The listing builds one solid part. Answer for the finished solid, in the listing's coordinates (mm). Face numbers are marked on the shaded views. A direction names the side the tool comes from. Round coordinates to 2 decimals unless told otherwise and drop trailing zeros. Write each loop counter-clockwise with the first axis right and the second up, starting at its lowest first coordinate (ties: lowest second). Pieces come first, ordered by that corner, then holes.
(1) A cutting plane is placed at A-A, the plane x = 0. Give the vertices of the cut face in (y, z) (3 decimals).
(2) A cutting plane is placed at B-B, the plane y = -16.5. Give the vertices of the cut face in (x, z).
(3) Each of these flat-tipped pins is pushed along its axis until it touches: pin 1 Ø3 at (y, z) = (0, 5) entering from +X (3 decimals); pin 2 Ø6 at (y, z) = (-4.5, 3) entering from -X; pin 3 Ø5.5 at (x, y) = (-9.9, -9.9) entering from +Z; pin 4 Ø2 at (x, y) = (9.9, -9.9) entering from +Z. Where does it stop, or does it pass through?
(4) For the marked faces 1, 2, 3 and 4, determine the directions among +Z, -Z, +X, -X, +Y, -Y from which every point of the face is accessible in a straight line to the end or side of a thin tool.
(5) Find the intervals of material crossed by probe 1 along Y at (x, z) = (0, 6.25) (3 decimals); probe 2 along X at (y, z) = (34.25, 5); probe 3 along X at (y, z) = (-34.5, 5), in increasing order.
(6) The mould has two halves that part along Z. Classify the marked faces 5, 6 and 7: +Z half, -Z half, draft (parallel to the pull), parting line (faces both ways), or undercut.
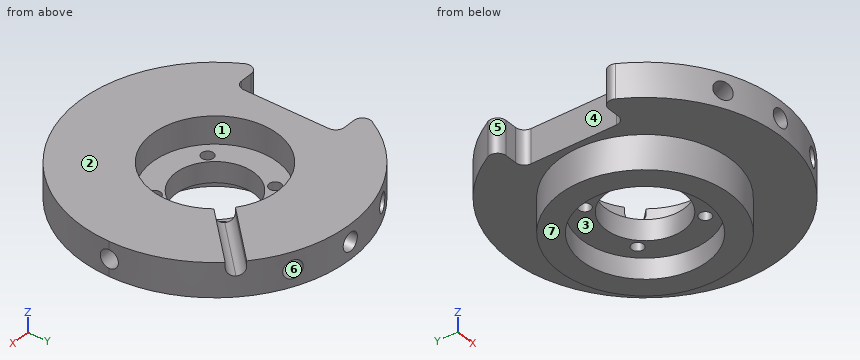
from build123d import *

# Parameters (mm, degrees)
SKETCH_1_R                = 39.675
EXTRUDE_1_DEPTH           = 10
SKETCH_7_R                = 2.65
CUT_EXTRUDE_5_DEPTH       = 8
PATTERN_CIRCULAR_1_COUNT  = 2
PATTERN_CIRCULAR_1_ANGLE  = 25
F_1_THE_OTHER_WAY_COUNT   = 2
F_1_THE_OTHER_WAY_ANGLE   = 25
MIRROR_1_COPY_1_SKETCH_R  = 2.65
MIRROR_1_COPY_1_DEPTH     = 8
MIRROR_1_COPY_2_SKETCH_R  = 2.65
MIRROR_1_COPY_2_DEPTH     = 8
SKETCH_9_R                = 2.65
CUT_EXTRUDE_7_DEPTH       = 8
PATTERN_CIRCULAR_2_COUNT  = 2
CUT_EXTRUDE_START         = -10
CUT_EXTRUDE_8_DEPTH       = 10
CUT_EXTRUDE_13_DEPTH      = 4
SKETCH_12_R               = 25
EXTRUDE_2_DEPTH           = 10
CUT_EXTRUDE_16_DEPTH      = 57.993080877
CUT_EXTRUDE_16_DEPTH_BACK = 57.993080877
SKETCH_18_R               = 11.5
SKETCH_18_R_2             = 1.75
SKETCH_19_R               = 18.4
CUT_EXTRUDE_17_DEPTH      = 6
CUT_EXTRUDE_START_2       = -8
SKETCH_20_R               = 18.4
CUT_EXTRUDE_18_DEPTH      = 8
FILLET_2_R                = 2.5


# Read off the part's stored shape, not the designer's step: Вырез-Вытянуть8
with BuildPart() as part:
    # Эскиз1 → Бобышка-Вытянуть1 (new body)
    with BuildSketch(Plane.XY):
        Circle(SKETCH_1_R)
    extrude(amount=EXTRUDE_1_DEPTH)

    # Эскиз7 → Вырез-Вытянуть5 (cut)
    with BuildSketch(Plane(origin=(0, 39.675, 0), x_dir=(0, 0, -1), z_dir=(0, 1, 0))):
        with Locations(Location((-5, 0, 0), (0, 0, 90))):
            Circle(SKETCH_7_R)
    cut_extrude_5 = extrude(amount=-CUT_EXTRUDE_5_DEPTH, mode=Mode.SUBTRACT)

    # Круговой массив1: Вырез-Вытянуть5 ×2 about axis
    pattern_circular_1_axis = Axis((0, 0, 10), (0, 0, -1))
    for i in range(1, PATTERN_CIRCULAR_1_COUNT):
        add(cut_extrude_5.rotate(pattern_circular_1_axis, i * PATTERN_CIRCULAR_1_ANGLE / (PATTERN_CIRCULAR_1_COUNT - 1)), mode=Mode.SUBTRACT)

    # 1 the other way: Вырез-Вытянуть5 ×2 about axis
    f_1_the_other_way_axis = Axis((0, 0, 10), (0, 0, 1))
    for i in range(1, F_1_THE_OTHER_WAY_COUNT):
        add(cut_extrude_5.rotate(f_1_the_other_way_axis, i * F_1_THE_OTHER_WAY_ANGLE / (F_1_THE_OTHER_WAY_COUNT - 1)), mode=Mode.SUBTRACT)

    # Зеркальное отражение1: Вырез-Вытянуть5 across plane
    add(cut_extrude_5.mirror(Plane.ZX), mode=Mode.SUBTRACT)

    # Зеркальное отражение1 copy 1 sketch → Зеркальное отражение1 copy 1 (cut)
    with BuildSketch(Plane(origin=(16.767379535, -35.957761451, 0), x_dir=(0, 0, -1), z_dir=(0.4226182617407035, -0.906307787036648, 0))):
        with Locations((-5, 0)):
            Circle(MIRROR_1_COPY_1_SKETCH_R)
    extrude(amount=-MIRROR_1_COPY_1_DEPTH, mode=Mode.SUBTRACT)

    # Зеркальное отражение1 copy 2 sketch → Зеркальное отражение1 copy 2 (cut)
    with BuildSketch(Plane(origin=(-16.767379535, -35.957761451, 0), x_dir=(0, 0, -1), z_dir=(-0.42261826174069717, -0.9063077870366509, 0))):
        with Locations((-5, 0)):
            Circle(MIRROR_1_COPY_2_SKETCH_R)
    extrude(amount=-MIRROR_1_COPY_2_DEPTH, mode=Mode.SUBTRACT)

    # Эскиз9 → Вырез-Вытянуть7 (cut)
    with BuildSketch(Plane.ZY.offset(39.675)):
        with Locations((5, 0)):
            Circle(SKETCH_9_R)
    cut_extrude_7 = extrude(amount=-CUT_EXTRUDE_7_DEPTH, mode=Mode.SUBTRACT)

    # Круговой массив2: Вырез-Вытянуть7 ×2 about axis
    pattern_circular_2_axis = Axis((0, 0, 10), (0, 0, -1))
    for i in range(1, PATTERN_CIRCULAR_2_COUNT):
        add(cut_extrude_7.rotate(pattern_circular_2_axis, i * 360 / PATTERN_CIRCULAR_2_COUNT), mode=Mode.SUBTRACT)

    # Вырез-Вытянуть8 outline → Вырез-Вытянуть8 (cut)
    with BuildSketch(Plane(origin=(0, 0, 0), x_dir=(-1, 0, 0), z_dir=(0, 0, -1)).offset(CUT_EXTRUDE_START)):
        with BuildLine():
            Line((36.730173223, 15), (26.730173223, 15))
            Line((26.730173223, 15), (26.730173223, -15))
            Line((26.730173223, -15), (36.730173223, -15))
            ThreePointArc((36.730173223, -15), (39.675, 0), (36.730173223, 15))
        make_face()
    extrude(amount=CUT_EXTRUDE_8_DEPTH, mode=Mode.SUBTRACT)

    # Эскиз15 → Вырез-Вытянуть13 (cut)
    with BuildSketch(Plane.XY.offset(10)):
        Polygon((-1.767766953, 1.767766953), (1.767766953, -1.767766953), (33.587572106, 30.0520382), (30.0520382, 33.587572106), align=None)
    extrude(amount=-CUT_EXTRUDE_13_DEPTH, mode=Mode.SUBTRACT)

    # Эскиз12 → Бобышка-Вытянуть2 (add)
    with BuildSketch(Plane.XY):
        Circle(SKETCH_12_R)
    extrude(amount=-EXTRUDE_2_DEPTH)

    # Эскиз18 → Вырез-Вытянуть16 (cut, two sides: drawn at the far end of the back side and taken through both)
    with BuildSketch(Plane(origin=(0, 0, 0), x_dir=(-1, 0, 0), z_dir=(0, 0, -1)).offset(-CUT_EXTRUDE_16_DEPTH_BACK)):
        Circle(SKETCH_18_R)
        with Locations((9.899494937, 9.899494937)):
            Circle(SKETCH_18_R_2)
        with Locations((9.899494937, -9.899494937)):
            Circle(SKETCH_18_R_2)
        with Locations((-9.899494937, -9.899494937)):
            Circle(SKETCH_18_R_2)
        with Locations((-9.899494937, 9.899494937)):
            Circle(SKETCH_18_R_2)
    extrude(amount=CUT_EXTRUDE_16_DEPTH + CUT_EXTRUDE_16_DEPTH_BACK, mode=Mode.SUBTRACT)

    # Эскиз19 → Вырез-Вытянуть17 (cut)
    with BuildSketch(Plane(origin=(0, 0, -10), x_dir=(-1, 0, 0), z_dir=(0, 0, -1))):
        Circle(SKETCH_19_R)
    extrude(amount=-CUT_EXTRUDE_17_DEPTH, mode=Mode.SUBTRACT)

    # Эскиз20 → Вырез-Вытянуть18 (cut)
    with BuildSketch(Plane.XY.offset(10).offset(CUT_EXTRUDE_START_2)):
        with Locations(Location((0, 0, 0), (0, 0, 180))):
            Circle(SKETCH_20_R)
    extrude(amount=CUT_EXTRUDE_18_DEPTH, mode=Mode.SUBTRACT)

    # Скругление2
    fillet_2_edges = [part.edges().sort_by_distance(p)[0] for p in [
        (18.676644746, 22.212178652, 6),
        (22.212178652, 18.676644746, 6),
        (-26.730173223, 15, 5),
        (-26.730173223, -15, 5),
    ]]
    fillet(fillet_2_edges, radius=FILLET_2_R - 0.0004)  # a hair under: the kernel refuses the full size
    fillet_2_2_edges = [part.edges().sort_by_distance(p)[0] for p in [
        (-36.730173223, -15, 5),
        (-36.730173223, 15, 5),
    ]]
    fillet(fillet_2_2_edges, radius=FILLET_2_R)


solid = part.part
Solutions:
1. outline: (-39.675, 0) - (-25, 0) - (-25, -10) - (-18.4, -10) - (-18.4, -4) - (-11.5, -4) - (-11.5, 2) - (-18.4, 2) - (-18.4, 10) - (-39.675, 10) - (-39.675, 7.65) - (-31.675, 7.65) - (-31.675, 2.35) - (-39.675, 2.35) - close; (11.5, -4) - (18.4, -4) - (18.4, -10) - (25, -10) - (25, 0) - (39.675, 0) - (39.675, 2.35) - (31.675, 2.35) - (31.675, 7.65) - (39.675, 7.65) - (39.675, 10) - (18.4, 10) - (18.4, 2) - (11.5, 2) - close
2. outline: (-35.09, 0) - (-18.78, 0) - (-18.78, -10) - (-8.14, -10) - (-8.14, -4) - (8.14, -4) - (8.14, -10) - (18.78, -10) - (18.78, 0) - (36.08, 0) - (36.08, 10) - (8.14, 10) - (8.14, 2) - (-8.14, 2) - (-8.14, 10) - (-35.09, 10) - close
3. pin 1: stops at x = 31.675
3. pin 2: stops at x = -26.73
3. pin 3: stops at z = 2
3. pin 4: passes through
4. face 1: +Z
4. face 2: +Z, +X, -X, +Y, -Y
4. face 3: -Z
4. face 4: +Z, -Z, -X
5. probe 1: y = -31.675 to -18.4, 18.4 to 31.675
5. probe 2: x = -20.03 to -18.89, -13.05 to -2.65, 2.65 to 13.05, 18.89 to 20.03
5. probe 3: x = -19.59 to -19.01, -13.16 to -2.65, 2.65 to 13.16, 19.01 to 19.59
6. face 5: draft
6. face 6: undercut
6. face 7: -Z half
